from build123d import *

# Parameters (mm, degrees)
SKETCH1_R               = 26.035
SKETCH1_R_2             = 23.495
BOSS_EXTRUDE1_DEPTH     = 12.7
CUT_EXTRUDE1_DEPTH      = 125.786790367
CUT_EXTRUDE1_DEPTH_BACK = 125.786790367


with BuildPart() as part:
    # Sketch1 → Boss-Extrude1 (new body)
    with BuildSketch(Plane(origin=(0, 0, 0), x_dir=(1, 0, 0), z_dir=(0, 1, 0))):
        with Locations(Location((-82.55, 0, 0), (0, 0, 270))):
            Circle(SKETCH1_R)
        with Locations(Location((-82.55, 0, 0), (0, 0, 270))):
            Circle(SKETCH1_R_2, mode=Mode.SUBTRACT)
    extrude(amount=BOSS_EXTRUDE1_DEPTH)

    # Sketch2 → Revolve1 (revolve)
    with BuildSketch(Plane(origin=(-82.55, 0, 0), x_dir=(0, -1, 0), z_dir=(-1, 0, 0)), mode=Mode.PRIVATE) as revolve1_sk:
        Polygon((0, -26.035), (0, -36.195), (-2.54, -36.195), (-12.7, -26.035), align=None)
    revolve(revolve1_sk.sketch.rotate(Axis((-82.55, 12.7, 0), (0, -1, 0)), 180), axis=Axis((-82.55, 12.7, 0), (0, -1, 0)))

    # Sketch3 → Cut-Extrude1 (cut, two sides: drawn at the far end of the back side and taken through both)
    with BuildSketch(Plane(origin=(0, 12.7, 0), x_dir=(1, 0, 0), z_dir=(0, 1, 0)).offset(-CUT_EXTRUDE1_DEPTH_BACK)):
        with BuildLine():
            ThreePointArc((-99.831769231, 31.802806122), (-104.775, 0), (-99.831769231, -31.802806122))
            ThreePointArc((-99.831769231, -31.802806122), (-118.745, 0), (-99.831769231, 31.802806122))
        make_face()
    extrude(amount=CUT_EXTRUDE1_DEPTH + CUT_EXTRUDE1_DEPTH_BACK, mode=Mode.SUBTRACT)


solid = part.part
Model file for the job. Use its own axes, mm. Round coordinates to 2 decimals unless told otherwise and drop trailing zeros. Loops run counter-clockwise (first coordinate to the right, second up) from the corner with the lowest first, then second, coordinate; pieces in that order, holes last.
1. Band-saw the part on A-A, the plane x = -82.55. List the corners of the cut face in (y, z) (3 decimals), and give its area (3 significant figures).
Check values:
outline: (0, -36.195) - (2.54, -36.195) - (12.7, -26.035) - (12.7, -23.495) - (0, -23.495) - close; (0, 23.495) - (12.7, 23.495) - (12.7, 26.035) - (2.54, 36.195) - (0, 36.195) - close
area: 219 mm2
2. Band-saw the part on B-B, the plane z = 0. List the corners of the cut face in (x, y) (3 decimals), and give its area (3 significant figures).
Check values:
outline: (-59.055, 0) - (-46.355, 0) - (-46.355, 2.54) - (-56.515, 12.7) - (-59.055, 12.7) - close
area: 110 mm2
3. Mould opens along Z. For faces 1 (the cylindrical face through (-103.236, 4.85, -17.892)), 2 (the flat face through (-56, 0, 1)), 3 (the cylindrical face through (-103.292, 4.85, 17.564)), 4 (the cylindrical face through (-59.073, 6.261, 0.91)) say: +Z half, -Z half, draft (parallel to the pull), parting line (faces both ways), or undercut.
Check values:
face 1: -Z half
face 2: draft
face 3: +Z half
face 4: undercut
4. Drop flat-ended pins along their axis: P1, Ø12, axis at x = -56.5, z = -27, coming from the +Y side; P2, Ø2, axis at y = 2.5, z = 4.5, coming from the +X side; P3, Ø4, axis at y = 9.5, z = -0.5, coming from the -X side. Give the stop position or say it passes through.
Check values:
P1: stops at y = 7.22
P2: stops at x = -46.52
P3: stops at x = -59.19
5. Wall check: probe 1 along Z at (x, y) = (-97, 5.25); probe 2 along Z at (x, y) = (-82.55, 4.5) (3 decimals); probe 3 along X at (y, z) = (7.75, -17). Give the ranges that are in metal, low to high.
Check values:
probe 1: z = -30.21 to -18.53, 18.53 to 30.21
probe 2: z = -34.235 to -23.495, 23.495 to 34.235
probe 3: x = -103.39 to -98.77, -66.33 to -56.64
